The figure shows three views and two pictorial views of one solid part (mm, origin at its lowest corner). Answer the questions. A direction names the side the tool comes from. Round coordinates to 2 decimals unless told otherwise and drop trailing zeros. Write each loop counter-clockwise with the first axis right and the second up, starting at its lowest first coordinate (ties: lowest second). Pieces come first, ordered by that corner, then holes.
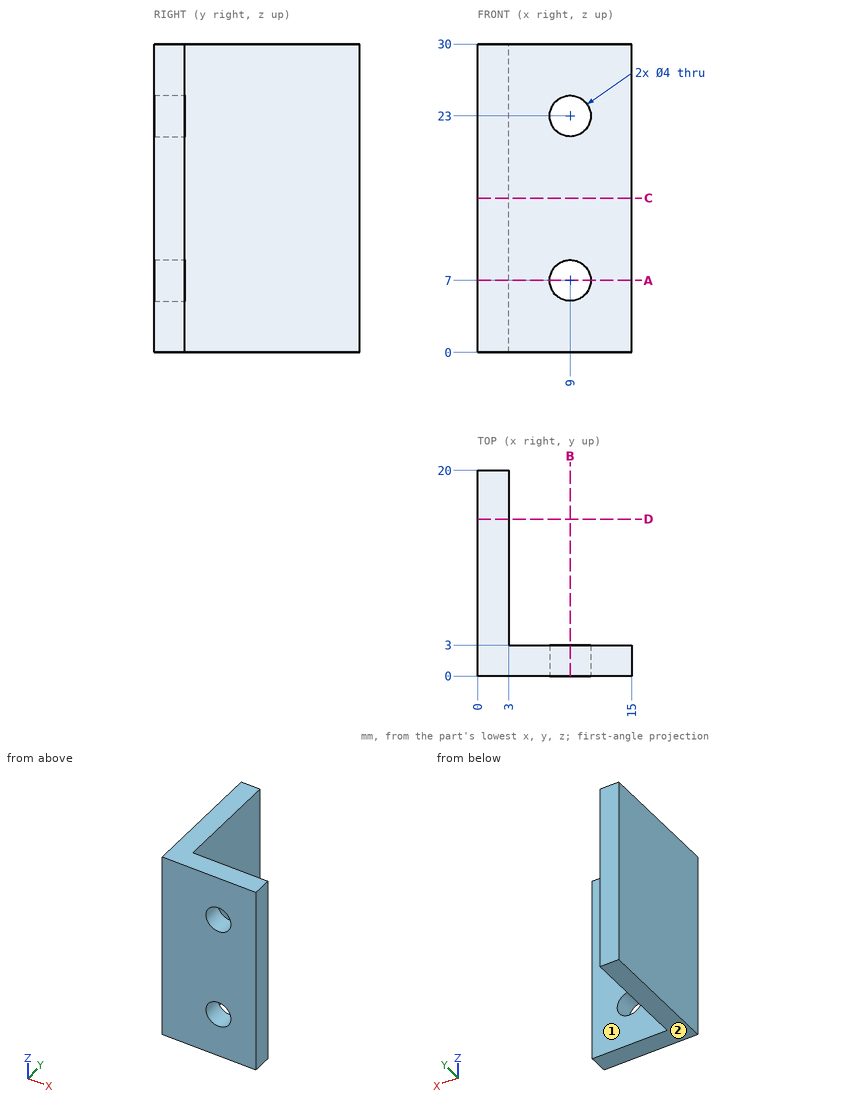
Q1. Section D-D (y = 15.25) is taken. Determine the outline of the cut face in (x, z), then the cut area to 3 significant figures.
Verdict:
outline: (0, 0) - (3, 0) - (3, 30) - (0, 30) - close
area: 90.0 mm2
Q2. Straight lines are drawn through the part: probe 1 along Z at (x, y) = (9, 1.5); probe 2 along X at (y, z) = (0.95, 23); probe 3 along Y at (x, z) = (12.75, 23.25). For each, find the intervals that lie inside material, in ascending order.
Verdict:
probe 1: z = 0 to 5, 9 to 21, 25 to 30
probe 2: x = 0 to 7, 11 to 15
probe 3: y = 0 to 3
Q3. Section B-B (x = 9) is taken. Determine the outline of the cut face in (y, z).
Verdict:
outline: (0, 0) - (3, 0) - (3, 5) - (0, 5) - close; (0, 9) - (3, 9) - (3, 21) - (0, 21) - close; (0, 25) - (3, 25) - (3, 30) - (0, 30) - close
Q4. Section A-A (z = 7) is taken. Determine the outline of the cut face in (x, y), then the cut area to 3 significant figures.
Verdict:
outline: (0, 0) - (7, 0) - (7, 3) - (3, 3) - (3, 20) - (0, 20) - close; (11, 0) - (15, 0) - (15, 3) - (11, 3) - close
area: 84.0 mm2
Q5. Section C-C (z = 15) is taken. Determine the outline of the cut face in (x, y), then the cut area to 3 significant figures.
Verdict:
outline: (0, 0) - (15, 0) - (15, 3) - (3, 3) - (3, 20) - (0, 20) - close
area: 96.0 mm2
Q6. Which of the six approach directions +Z, -Z, +X, -X, +Y, -Y give full straight-line access (tool end or side, diameter ignored) to the marked faces 1 and 2?
Verdict:
face 1: +Z, -Z, +X, +Y
face 2: -Z, +X, -X, +Y, -Y
Q7. Flat-ended cylindrical pins translate along their axes: pin 1 Ø10 at (y, z) = (13, 3.5) entering from +X; pin 2 Ø1 at (x, z) = (4, 14.5) entering from +Y. Find the tip coordinate at first contact, or state that the pin passes through.
Verdict:
pin 1: stops at x = 3
pin 2: stops at y = 3
